Could you check a few things on this model? Use its own coordinates, in mm. A direction names the side the tool comes from. Coordinates: 2 decimals unless noted, no trailing zeros. Loops run counter-clockwise (first coordinate to the right, second up) from the corner with the lowest first, then second, coordinate; pieces in that order, holes last.
1) Imagine slicing it at C-C on z = 9. Please give me the cut outline in (x, y), plus the area to 3 significant figures.
2) For faces 4 (the face through (79, 64, -20)), 5 (the face through (109.696, 40.425, 19.72)), 6 (the face through (15.773, 17.32, -9.86)), which set-ups out of +Z, -Z, +X, -X, +Y, -Y let a thin tool reach every point of the face, with its end or its side?
3) Thinking about a two-plate mould opening in X: for faces 1 (the face through (96.4, 46.9, 0)), 2 (the face through (34.131, 90.466, -9.86)), 3 (the face through (50, 64, 0)), which applies, released by +X, released by -X, zero draft, split by the parting line, or undercut?
4) If I drill on line 1 along Y through (x, z) = (0, -8.5); line 2 along Y through (x, z) = (-27.5, -12); line 3 along Z through (x, y) = (109, 135.5), over which ranges is the centre line in solid material (lowest first)?
5) Imagine slicing it at D-D on y = 132.5. Please give me the cut outline in (x, z), plus the area to 3 significant figures.
6) Imagine slicing it at A-A on z = -8.5. Please give me the cut outline in (x, y), plus the area to 3 significant figures.
7) Imagine slicing it at B-B on x = 82.5. Please give me the cut outline in (y, z).
8) Will these pins go through, and if not, where does the flat tip stop? P1, Ø12, axis at x = 0, y = 0, coming from the +Z side; P2, Ø10, axis at x = -25.5, z = -8, coming from the +Y side; P3, Ø15, axis at x = 79.5, y = 44, coming from the +Z side; P4, Ø10, axis at x = -25.5, z = -11, coming from the -Y side.
```python
from build123d import *

# Parameters (mm, degrees)
F0_R      = 25
F0_R_2    = 17.5
F0_R_3    = 7.5
F1_DEPTH  = 20
F2_DEPTH  = 40
F3_R      = 15
F4_DEPTH  = 40
F5_R      = 10
F6_DEPTH  = 20
F7_R      = 15
F8_DEPTH  = 20.001
F9_R      = 17.5
F10_DEPTH = 3


with BuildPart() as f1:
    # F0 (on Top) → F1 (new body)
    with BuildSketch(Plane.XY):
        with BuildLine():
            ThreePointArc((61.9906852191, 154.3882326301), (33.5268459232, 89.6702692228), (-21.4201114342, 45.1794071026))
            ThreePointArc((-21.4201114342, 45.1794071026), (-45.7124014002, -20.2577481036), (19.0821348166, -46.2154966525))
            Line((19.0821348166, -46.2154966525), (196.1436077868, 26.8922516737))
            ThreePointArc((196.1436077868, 26.8922516737), (161.7368914415, 47.4116601952), (191.1799201156, 74.5773797371))
            ThreePointArc((191.1799201156, 74.5773797371), (138.7787609454, 102.1762205669), (111.1799201156, 154.5773797371))
            ThreePointArc((111.1799201156, 154.5773797371), (111.4966611043, 152.2984240875), (111.6025403784, 150))
            ThreePointArc((111.6025403784, 150), (84.3998578075, 125.0972252652), (61.9906852191, 154.3882326301))
        make_face()
        with BuildLine():
            ThreePointArc((21.6506350946, 27.5), (31.4862845403, 15.2844327943), (35, 0))
            ThreePointArc((35, 0), (31.4862845403, -15.2844327943), (21.6506350946, -27.5))
            ThreePointArc((21.6506350946, -27.5), (17.5, -30.3108891325), (12.9903810568, -32.5))
            ThreePointArc((12.9903810568, -32.5), (-17.5, -30.3108891325), (-34.6410161514, -5))
            ThreePointArc((-34.6410161514, -5), (-35, 0), (-34.6410161514, 5))
            ThreePointArc((-34.6410161514, 5), (-17.5, 30.3108891325), (12.9903810568, 32.5))
            ThreePointArc((12.9903810568, 32.5), (17.5, 30.3108891325), (21.6506350946, 27.5))
        make_face(mode=Mode.SUBTRACT)
        with Locations((86.6025403784, 50)):
            Circle(F0_R, mode=Mode.SUBTRACT)
        with BuildLine():
            ThreePointArc((191.1799201156, 74.5773797371), (161.7368914415, 47.4116601952), (196.1436077868, 26.8922516737))
            ThreePointArc((196.1436077868, 26.8922516737), (207.3814561972, 36.0990411339), (211.6025403784, 50))
            ThreePointArc((211.6025403784, 50), (205.8305732137, 65.9775703186), (191.1799201156, 74.5773797371))
        make_face()
        with Locations((186.6025403784, 50)):
            Circle(F0_R_2, mode=Mode.SUBTRACT)
        with BuildLine():
            ThreePointArc((111.1799201156, 154.5773797371), (86.5064087202, 174.9998151734), (61.9906852191, 154.3882326301))
            ThreePointArc((61.9906852191, 154.3882326301), (84.3998578075, 125.0972252652), (111.6025403784, 150))
            ThreePointArc((111.6025403784, 150), (111.4966611043, 152.2984240875), (111.1799201156, 154.5773797371))
        make_face()
        with Locations((86.6025403784, 150)):
            Circle(F0_R_2, mode=Mode.SUBTRACT)
        with Locations((86.6025403784, 50)):
            Circle(F0_R)
        with Locations((186.6025403784, 50)):
            Circle(F0_R_2)
        with Locations((86.6025403784, 150)):
            Circle(F0_R_2)
        with BuildLine():
            ThreePointArc((12.5, 0), (11.8739069596, 3.9064476849), (10.0583466376, 7.4215674165))
            ThreePointArc((10.0583466376, 7.4215674165), (6.25, 10.8253175473), (1.3980925998, 12.4215674165))
            ThreePointArc((1.3980925998, 12.4215674165), (-6.25, 10.8253175473), (-11.4564392374, 5))
            ThreePointArc((-11.4564392374, 5), (-12.5, 0), (-11.4564392374, -5))
            ThreePointArc((-11.4564392374, -5), (-6.25, -10.8253175473), (1.3980925998, -12.4215674165))
            ThreePointArc((1.3980925998, -12.4215674165), (6.25, -10.8253175473), (10.0583466376, -7.4215674165))
            ThreePointArc((10.0583466376, -7.4215674165), (11.8739069596, -3.9064476849), (12.5, 0))
        make_face()
        Circle(F0_R_3, mode=Mode.SUBTRACT)
        with BuildLine():
            Line((10.0583466376, 7.4215674165), (21.6506350946, 27.5))
            ThreePointArc((21.6506350946, 27.5), (17.5, 30.3108891325), (12.9903810568, 32.5))
            Line((12.9903810568, 32.5), (1.3980925998, 12.4215674165))
            ThreePointArc((1.3980925998, 12.4215674165), (6.25, 10.8253175473), (10.0583466376, 7.4215674165))
        make_face()
        with BuildLine():
            Line((-11.4564392374, 5), (-34.6410161514, 5))
            ThreePointArc((-34.6410161514, 5), (-35, 0), (-34.6410161514, -5))
            Line((-34.6410161514, -5), (-11.4564392374, -5))
            ThreePointArc((-11.4564392374, -5), (-12.5, 0), (-11.4564392374, 5))
        make_face()
        with BuildLine():
            ThreePointArc((12.9903810568, -32.5), (17.5, -30.3108891325), (21.6506350946, -27.5))
            Line((21.6506350946, -27.5), (10.0583466376, -7.4215674165))
            ThreePointArc((10.0583466376, -7.4215674165), (6.25, -10.8253175473), (1.3980925998, -12.4215674165))
            Line((1.3980925998, -12.4215674165), (12.9903810568, -32.5))
        make_face()
    extrude(amount=-F1_DEPTH)

    # F0 (on Top) → F2 (join)
    with BuildSketch(Plane.XY):
        with Locations((86.6025403784, 50)):
            Circle(F0_R)
    extrude(amount=F2_DEPTH)

    # F3 (on face) → F4 (cut, through all)
    with BuildSketch(Plane.XY.offset(40)):
        with Locations((86.6025403784, 50)):
            Circle(F3_R)
    extrude(amount=-F4_DEPTH, mode=Mode.SUBTRACT)

    # F5 (on face) → F6 (cut, through all)
    with BuildSketch(Plane(origin=(0, 0, -20), x_dir=(1, 0, 0), z_dir=(0, 0, -1))):
        with Locations((86.6025403784, -50)):
            Circle(F5_R)
    extrude(amount=-F6_DEPTH, mode=Mode.SUBTRACT)

    # F7 (on face) → F8 (cut, through all)
    with BuildSketch(Plane.XY):
        with Locations((186.6025403784, 50)):
            Circle(F7_R)
    extrude(amount=-F8_DEPTH, mode=Mode.SUBTRACT)

    # F9 (on face) → F10 (cut)
    with BuildSketch(Plane.XY):
        with Locations((186.6025403784, 50)):
            Circle(F9_R)
    extrude(amount=-F10_DEPTH, mode=Mode.SUBTRACT)


solid = f1.part
```
Filled in:
1. outline: circle Ø50 at (86.6, 50); hole circle Ø30 at (86.6, 50)
1. area: 1,260 mm2
2. face 4: -Z, +X, -X, +Y, -Y
2. face 5: +Z
2. face 6: +Z, -Z
3. face 1: undercut
3. face 2: released by -X
3. face 3: zero draft
4. line 1: y = -50 to -35, -12.5 to -7.5, 7.5 to 12.5, 35 to 57.6
4. line 2: y = -41.76 to -21.65, -5 to 5, 21.65 to 41.76
4. line 3: z = -20 to 0
5. outline: (56.36, -20) - (118.01, -20) - (118.01, 0) - (56.36, 0) - close
5. area: 1,230 mm2
6. outline: (-21.42, 45.18) arc R50 ccw to (19.08, -46.22) - (196.14, 26.89) arc R25 ccw to (191.18, 74.58) arc R100 cw to (111.18, 154.58) arc R25 ccw to (61.99, 154.39) arc R150 cw to start; hole (-34.64, -5) arc R35 ccw to (12.99, -32.5) - (1.4, -12.42) arc R12.5 cw to (-11.46, -5) - close; hole (-34.64, 5) - (-11.46, 5) arc R12.5 cw to (1.4, 12.42) - (12.99, 32.5) arc R35 ccw to start; hole circle Ø15 at (0, 0); hole (10.06, -7.42) - (21.65, -27.5) arc R35 ccw to (21.65, 27.5) - (10.06, 7.42) arc R12.5 cw to start; hole circle Ø20 at (86.6, 50); hole circle Ø30 at (186.6, 50)
6. area: 25,500 mm2
7. outline: (-20.03, -20) - (40.88, -20) - (40.88, 0) - (35.57, 0) - (35.57, 40) - (25.34, 40) - (25.34, 0) - (-20.03, 0) - close; (59.12, -20) - (174.66, -20) - (174.66, 0) - (74.66, 0) - (74.66, 40) - (64.43, 40) - (64.43, 0) - (59.12, 0) - close
8. P1: passes through
8. P2: stops at y = 45.62
8. P3: stops at z = 40
8. P4: stops at y = -45.6
